Verification items for the finished model (mm, model axes). Face numbers are marked on the shaded views. A direction names the side the tool comes from. Coordinates: 2 decimals unless noted, no trailing zeros. Order: outer loops, then holes, each group sorted by start corner. A loop starts at its lowest first (then second) coordinate and runs counter-clockwise, first axis right, second up. Notation, with made-up numbers: M 44,56 L 53,56 A7 ccw 53,65 Z; hole C 78,34 d11. An arc over 180 degrees is marked long. Return JSON: item names as keys, results as strings. Group by question number.
1. Section check A-A, the plane y = -8.55. Record the cut outline in (x, z), plus the area to 3 significant figures.
2. Set-up check for the marked faces 1, 2, 3, 4 and 5: record each of +Z, -Z, +X, -X, +Y, -Y from which the full face is reachable in a straight line by a thin tool's end or side.
3. Material ranges on line 1 along X through (y, z) = (-10.3, -7.5); line 2 along Y through (x, z) = (0, 16); line 3 along Z through (x, y) = (-21, -10.2), recorded low to high.
4. Section check D-D, the plane x = 7. Record the cut outline in (y, z), plus the area to 3 significant figures.
5. Gauge pin test, flat ends, axial feed: pin 1 (6 mm diameter, centred on y = 5, z = -4.5, fed in from +X); pin 2 (4.5 mm diameter, centred on x = 7.4, y = 4.28, fed in from -Z); pin 3 (6 mm diameter, centred on x = 7, z = 3.5, fed in from +Y) (3 decimals); pin 4 (1.7 mm diameter, centred on x = 0, y = 8.55, fed in from -Z). Record the tip position at first contact, or that the pin passes through.
6. Section check C-C, the plane x = 21. Record the cut outline in (y, z), plus the area to 3 significant figures.
7. Section check B-B, the plane z = -7.5. Record the cut outline in (x, y).
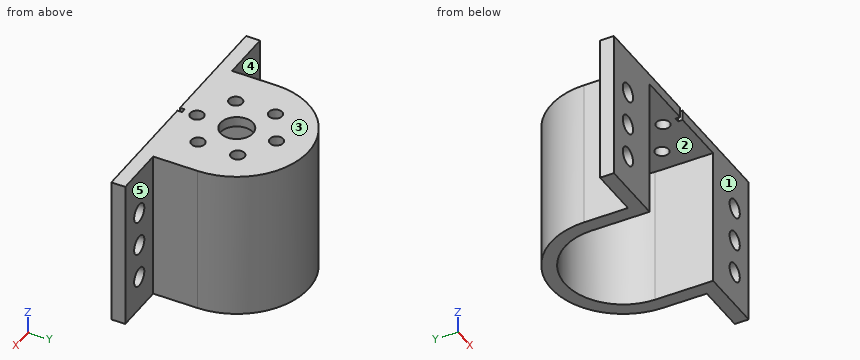
Autodesk Inventor part; units mm, degrees
ref_plane "YZ Plane" through (0, 0, 0) normal (1, 0, 0) x (0, 1, 0)
ref_plane "XZ Plane" through (0, 0, 0) normal (0, 1, 0) x (-1, 0, 0)
ref_plane "XY Plane" through (0, 0, 0) normal (0, 0, 1) x (1, 0, 0)
sketch "Эскиз1" plane through (0, 0, 0) normal (0, 0, 1) x (1, 0, 0)
  arc A0 (12.5, 0) -> (-12.5, 0) centre (0, 0) ccw
  line L0 (-14, -15) -> (14, 15) construction
  line L1 (14, -15) -> (-14, 15) construction
  line L2 (-14, 0) -> (14, 0) construction
  line L3 (-12.5, 0) -> (-12.5, -12.5)
  line L4 (12.5, 0) -> (12.5, -12.5)
  line L5 (-14, -12.5) -> (-12.5, -12.5)
  line L6 (12.5, -12.5) -> (14, -12.5)
  arc A1 (-12.5, 0) -> (12.5, 0) centre (0, 0) ccw construction
  line L7 (-16.5, 17.6786) -> (16.5, -17.6786) construction
  line L8 (16.5, 17.6786) -> (-16.5, -17.6786) construction
  line L9 (-16.5, -12.5) -> (-12.5, -12.5)
  line L10 (12.5, -12.5) -> (16.5, -12.5)
  arc A2 (-12.2571, 13.1326) -> (-12.5, 12.8766) centre (-1.5, 2.6786) ccw
  line L11 (16.5, -12.5) -> (26.5, -12.5)
  line L12 (0, 24.347) -> (0, -20.4254) construction
  line L13 (-16.5, -12.5) -> (-26.5, -12.5)
  line L14 (-15.5, -9.5) -> (-15.5, 0)
  arc A3 (15.5, 0) -> (-15.5, 0) centre (0, 0) ccw
  line L15 (15.5, 0) -> (15.5, -9.5)
  line L16 (-12.5, -12.5) -> (-12.5, -9.5)
  line L17 (-26.5, -12.5) -> (-12.5, -12.5)
  line L18 (-12.5, -12.5) -> (-12.5, -9.5)
  line L19 (-15.5, -9.5) -> (-26.5, -9.5)
  line L20 (-26.5, -9.5) -> (-26.5, -12.5)
  line L21 (12.5, -12.5) -> (26.5, -12.5)
  line L22 (26.5, -12.5) -> (26.5, -9.5)
  line L23 (26.5, -9.5) -> (15.5, -9.5)
  line L24 (12.5, -9.5) -> (12.5, -12.5)
  point P0 (0, 17.6786)
  dimension "d0" = 25
  dimension "d5" = 15
  dimension "d38" = 3
  dimension "d39" = 3
extrude "Выдавливание1" add sketch "Эскиз1" along normal mid plane 30
sketch "Эскиз7" plane through (-26.5, -9.5, 15) normal (0, 1, 0) x (1, 0, 0)
  line L0 (0, 15) -> (11, 15) construction
  line L1 (11, 30) -> (11, 0) construction
  line L2 (5.5, 0) -> (5.5, 30) construction
  line L3 (0, 30) -> (11, 30) construction
  line L4 (0, 7.5) -> (11, 7.5) construction
  line L5 (0, 22.5) -> (11, 22.5) construction
  circle A0 centre (5.5, 7.5) radius 2
  line L6 (0, 0) -> (0, 30)
  line L7 (0, 30) -> (0, 0)
  circle A1 centre (5.5, 15) radius 2
  circle A2 centre (5.5, 22.5) radius 2
  line L8 (26.5, 38.2442) -> (26.5, 0)
  line L9 (53, 15) -> (42, 15) construction
  line L10 (42, 30) -> (42, 0) construction
  line L11 (47.5, 0) -> (47.5, 30) construction
  line L12 (53, 30) -> (42, 30) construction
  line L13 (53, 7.5) -> (42, 7.5) construction
  line L14 (53, 22.5) -> (42, 22.5) construction
  circle A3 centre (47.5, 7.5) radius 2
  circle A4 centre (47.5, 15) radius 2
  circle A5 centre (47.5, 22.5) radius 2
  point P0 (26.5, 15)
  dimension "d40" = 4
  dimension "d41" = 4
  dimension "d42" = 4
extrude "Выдавливание7" cut sketch "Эскиз7" against normal blind 10
sketch "Эскиз8" plane through (0, 0, 15) normal (0, 0, 1) x (1, 0, 0)
  line L0 (-15.5, -9.5) -> (15.5, -9.5)
split_face "Разделение1"
sketch "Эскиз9" plane through (0, 0, 15) normal (0, 0, 1) x (1, 0, 0)
  arc A0 (15.5, 0) -> (-15.5, 0) centre (0, 0) ccw
  line L0 (-15.5, 0) -> (-15.5, -9.5)
  line L1 (15.5, 0) -> (15.5, -9.5)
  line L2 (12.5, -12.5) -> (26.5, -12.5)
  line L3 (-15.5, -9.5) -> (-26.5, -9.5)
  line L4 (-26.5, -9.5) -> (-26.5, -12.5)
  line L5 (-26.5, -12.5) -> (-12.5, -12.5)
  line L6 (15.5, -9.5) -> (26.5, -9.5)
  line L7 (26.5, -9.5) -> (26.5, -12.5)
  line L8 (-12.5, -12.5) -> (12.5, -12.5)
  point P0 (-12.5, 0)
  point P1 (12.5, 0)
  point P2 (-12.5, -9.5)
extrude "Выдавливание8" add sketch "Эскиз9" along normal blind 2.2
sketch "Эскиз10" plane through (0, 0, 17.2) normal (0, 0, 1) x (1, 0, 0)
  arc A0 (12.5, 0) -> (-12.5, 0) centre (0, 0) ccw
  line L0 (12.5, 0) -> (12.5, -12.5)
  line L1 (-12.5, -12.5) -> (-12.5, 0)
  circle A1 centre (0, 0) radius 12.5 construction
  circle A2 centre (0, 0) radius 3.5
  line L2 (0, 12.5) -> (0, 10) construction
  line L3 (0, 10) -> (0, 7.1) construction
  circle A3 centre (0, 8.55) radius 1.45
  line L4 (-12.5, 0) -> (12.5, 0) construction
  circle A4 centre (-7.4045, 4.275) radius 1.45
  circle A5 centre (-7.4045, -4.275) radius 1.45
  circle A6 centre (0, -8.55) radius 1.45
  circle A7 centre (7.4045, -4.275) radius 1.45
  circle A8 centre (7.4045, 4.275) radius 1.45
  point P0 (-8.6603, 5)
  point P1 (-8.6603, -5)
  point P2 (0, -10)
  point P3 (8.6603, -5)
  point P4 (8.6603, 5)
  dimension "d47" = 7
  dimension "d48" = 2.5
  dimension "d49" = 2.9
  dimension "d52" = 360
extrude "Выдавливание9" cut sketch "Эскиз10" against normal blind 3
sketch "Эскиз11" plane through (-26.5, -12.5, -15) normal (0, -1, 0) x (1, 0, 0)
  line L0 (0, 32.2) -> (53, 32.2)
  line L1 (26.5, 32.2) -> (26.5, 30)
  line L2 (30, 30) -> (23, 30)
  line L3 (27, 30) -> (26, 30)
  line L4 (26, 30) -> (26, 32.2)
  line L5 (26, 32.2) -> (27, 32.2)
  line L6 (27, 32.2) -> (27, 30)
  line L7 (27, 30) -> (26, 32.2) construction
  line L8 (26, 30) -> (27, 32.2) construction
  point P0 (26.5, 15)
  point P1 (26.5, 31.1)
  dimension "d56" = 1
extrude "Выдавливание10" cut sketch "Эскиз11" against normal blind 1
sketch "Эскиз12" plane through (0, 0, 17.2) normal (0, 0, 1) x (1, 0, 0)
  arc A0 (15.5, 0) -> (-15.5, 0) centre (0, 0) ccw construction
  line L0 (0, 15.5) -> (0, -12.7683) construction
properties part number "Mount gor motor TR"
Answers follow:
{
 "1": {"outline": "M -15.5,-15 L -12.5,-15 L -12.5,15 L -1.45,15 L -1.45,17.2 L -15.5,17.2 Z; M 1.45,15 L 12.5,15 L 12.5,-15 L 15.5,-15 L 15.5,17.2 L 1.45,17.2 Z", "area": "242 mm^2"},
 "2": {"face 1": "+Z, -Z, +X, -X, -Y", "face 2": "-Z, -Y", "face 3": "+Z, +X, -X, +Y, -Y", "face 4": "+Z, -Z, -X, +Y", "face 5": "+Z, -Z, +X, +Y"},
 "3": {"line 1": "-26.5 to -23, -19 to -12.5, 12.5 to 19, 23 to 26.5", "line 2": "-11.5 to -10, -7.1 to -3.5, 3.5 to 7.1, 10 to 15.5", "line 3": "-15 to -9.5, -5.5 to -2, 2 to 5.5, 9.5 to 17.2"},
 "4": {"outline": "M -12.5,15 L -5.67,15 L -5.67,17.2 L -12.5,17.2 Z; M -2.88,15 L 2.88,15 L 2.88,17.2 L -2.88,17.2 Z; M 5.67,15 L 10.36,15 L 10.36,-15 L 13.83,-15 L 13.83,17.2 L 5.67,17.2 Z", "area": "150 mm^2"},
 "5": {"pin 1": "x = 15.37", "pin 2": "z = 15", "pin 3": "y = 14.975", "pin 4": "through"},
 "6": {"outline": "M -12.5,-15 L -9.5,-15 L -9.5,-9.5 L -12.5,-9.5 Z; M -12.5,-5.5 L -9.5,-5.5 L -9.5,-2 L -12.5,-2 Z; M -12.5,2 L -9.5,2 L -9.5,5.5 L -12.5,5.5 Z; M -12.5,9.5 L -9.5,9.5 L -9.5,17.2 L -12.5,17.2 Z", "area": "60.6 mm^2"},
 "7": {"outline": "M -26.5,-12.5 L -23,-12.5 L -23,-9.5 L -26.5,-9.5 Z; M -19,-12.5 L -12.5,-12.5 L -12.5,0 A12.5 cw 12.5,0 L 12.5,-12.5 L 19,-12.5 L 19,-9.5 L 15.5,-9.5 L 15.5,0 A15.5 ccw -15.5,0 L -15.5,-9.5 L -19,-9.5 Z; M 23,-12.5 L 26.5,-12.5 L 26.5,-9.5 L 23,-9.5 Z"}
}
